The listing builds one solid part. Answer for the finished solid, in the listing's coordinates (mm). Give positions to 0.01 mm unless a question says otherwise; leave off trailing zeros. Write each loop counter-clockwise with the first axis right and the second up, starting at its lowest first coordinate (ties: lowest second). Pieces come first, ordered by that corner, then holes. Notation, with made-up numbers: M 40,47.25 L 67,47.25 A6 ccw 67,57.25 Z; hole C 2.25,-7.75 d8. An arc over 180 degrees is marked long. Return JSON: item names as keys, results as strings.
from build123d import *

# Parameters (mm, degrees)
SKETCH_1_W          = 420
SKETCH_1_H          = 550
EXTRUDE_1_DEPTH     = 5
SKETCH_2_R          = 2.5
CUT_EXTRUDE_1_DEPTH = 15
FILLET_1_R          = 5


with BuildPart() as part:
    # 草图1 → 凸台-拉伸1 (new body)
    with BuildSketch(Plane.XY):
        Rectangle(SKETCH_1_W, SKETCH_1_H)
    extrude(amount=EXTRUDE_1_DEPTH)

    # 草图2 → 切除-拉伸1 (cut)
    with BuildSketch(Plane.XY.offset(5)):
        with Locations((-200, 195)):
            Circle(SKETCH_2_R)
        with Locations((-140, 265)):
            Circle(SKETCH_2_R)
        with Locations((-140, -265)):
            Circle(SKETCH_2_R)
        with Locations((-140, -145)):
            Circle(SKETCH_2_R)
        with Locations((-200, -125)):
            Circle(SKETCH_2_R)
        with Locations((200, 265)):
            Circle(SKETCH_2_R)
        with Locations((200, -265)):
            Circle(SKETCH_2_R)
        Polygon((-190, 255), (-190, 215), (-210, 215), (-210, 275), (-150, 275), (-150, 255), align=None)
        Polygon((-190, -255), (-150, -255), (-150, -275), (-210, -275), (-210, -135), (-150, -135), (-150, -155), (-190, -155), align=None)
    extrude(amount=-CUT_EXTRUDE_1_DEPTH, mode=Mode.SUBTRACT)

    # 圆角1
    fillet_1_edges = [part.edges().sort_by_distance(p)[0] for p in [
        (-210, -135, 2.5),
        (-150, -135, 2.5),
        (-150, -155, 2.5),
        (-190, -155, 2.5),
        (-190, -255, 2.5),
        (-150, -255, 2.5),
        (-150, -275, 2.5),
        (-150, 275, 2.5),
        (-150, 255, 2.5),
        (-190, 255, 2.5),
        (-190, 215, 2.5),
        (-210, 215, 2.5),
        (210, -275, 2.5),
        (210, 275, 2.5),
    ]]
    fillet(fillet_1_edges, radius=FILLET_1_R)


solid = part.part
Item 1: A cutting plane is placed at B-B, the plane y = -218. Write down the section's boundary in (x, z), plus the area to 3 significant figures.
Geometry results:
{"outline": "M -190,0 L 210,0 L 210,5 L -190,5 Z", "area": "2,000 mm2"}
Item 2: A cutting plane is placed at A-A, the plane z = 3.5. Count the separate pieces of the cut face and the enclosed holes in it, plus the area to 3 significant figures.
Geometry results:
{"separate pieces": "1", "enclosed holes": "7", "area": "224,000 mm2"}
Item 3: Given pin 1 Ø4.5 at (x, y) = (-140, -145) entering from -Z; pin 2 Ø2.5 at (y, z) = (267, 3) entering from -X; pin 3 Ø8 at (x, y) = (200, 265) entering from -Z, each flat-ended and moving along its own axis, determine where each tip first touches the part or whether it passes through.
Geometry results:
{"pin 1": "passes through", "pin 2": "stops at x = -150", "pin 3": "stops at z = 0"}
Item 4: Find the intervals of material crossed by line 1 (X direction, y = 265, z = 3.6); line 2 (Y direction, x = 200, z = 1.8); line 3 (Y direction, x = -140, z = 1.3), in increasing order.
Geometry results:
{"line 1": "x = -150 to -142.5, -137.5 to 197.5, 202.5 to 210", "line 2": "y = -275 to -267.5, -262.5 to 262.5, 267.5 to 275", "line 3": "y = -275 to -267.5, -262.5 to -147.5, -142.5 to 262.5, 267.5 to 275"}
